Study the drawing (mm; zero at the part's minimum x, y, z) and answer. A direction names the side the tool comes from. Give positions to 0.01 mm unless a question says otherwise; leave off trailing zeros. Loops run counter-clockwise (first coordinate to the right, second up) from the corner with the lowest first, then second, coordinate; pieces in that order, holes last. Notation, with made-up numbers: M 66,-30 L 92,-30 A18 cw 92,-7 Z; hole C 33,53.25 d5. An arc over 180 degrees is marked long. Return JSON: item names as keys, results as strings.
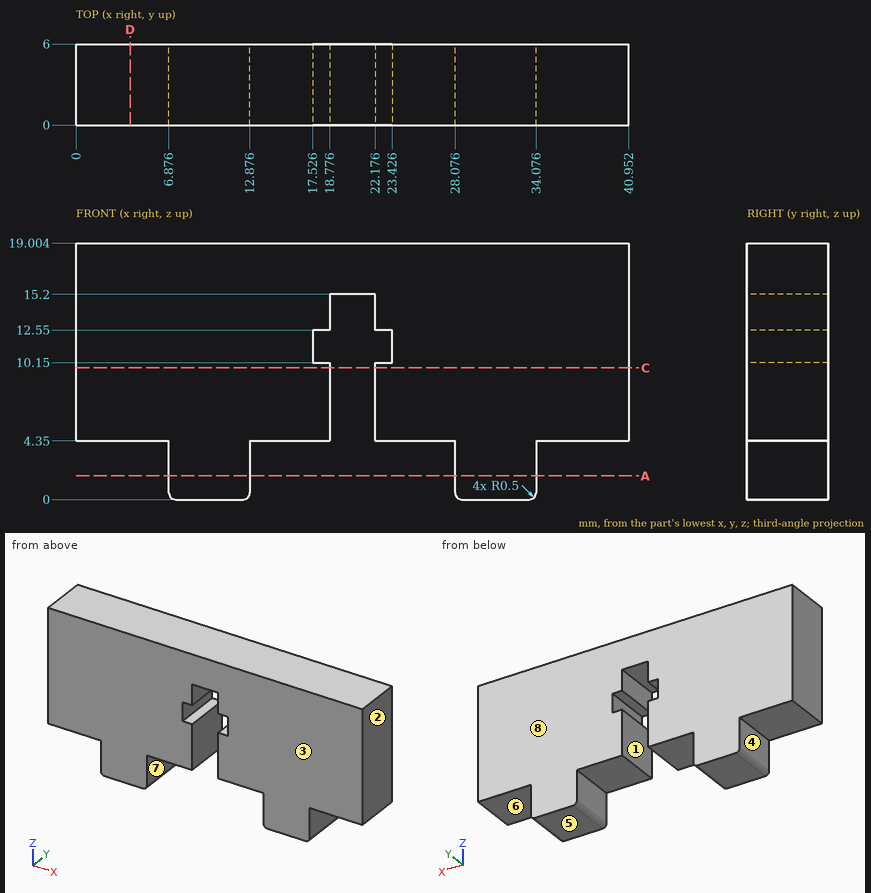
(1) The part is cut by section C-C (z = 9.75). Determine the outline of the cut face in (x, y) (1 decimal), and give its area (3 significant figures).
Values follow:
{"outline": "M 0,0 L 18.8,0 L 18.8,6 L 0,6 Z; M 22.2,0 L 41,0 L 41,6 L 22.2,6 Z", "area": "225 mm²"}
(2) Given pin 1 (1.5 mm diameter, centred on x = 5.5, z = 3, fed in from +Y); pin 2 (1.4 mm diameter, centred on x = 18, y = 2.5, fed in from -Z); pin 3 (1.2 mm diameter, centred on y = 4, z = 2, fed in from +X), each flat-ended and moving along its own axis, determine where each tip first touches the part or whether it passes through.
Values follow:
{"pin 1": "through", "pin 2": "z = 4.35", "pin 3": "x = 34.08"}
(3) A tool of negligible diameter and unlimited length cuts with its end or side. For the marked faces 4, 5, 6, 7 and 8, from which of +Z, -Z, +X, -X, +Y, -Y can it reach the whole face along a straight path? Write none if from no direction.
Values follow:
{"face 4": "-Z, -X, +Y, -Y", "face 5": "-Z, +X, -X, +Y, -Y", "face 6": "-Z, +X, +Y, -Y", "face 7": "-Z, +Y, -Y", "face 8": "+Z, -Z, +X, -X, +Y"}
(4) The part is cut by section D-D (x = 4). Determine the outline of the cut face in (y, z).
Values follow:
{"outline": "M 0,4.35 L 6,4.35 L 6,19 L 0,19 Z"}
(5) Straight lines are drawn through the part: line 1 along X through (y, z) = (1.45, 3.75) (1 decimal); line 2 along X through (y, z) = (1.5, 10.75) (1 decimal); line 3 along Z through (x, y) = (22.5, 1.25). For each, find the intervals that lie inside material, in ascending order.
Values follow:
{"line 1": "6.9 to 12.9, 28.1 to 34.1", "line 2": "0 to 17.5, 23.4 to 41", "line 3": "4.35 to 10.15, 12.55 to 19"}
(6) The part is cut by section A-A (z = 1.75). Determine the outline of the cut face in (x, y) (1 decimal).
Values follow:
{"outline": "M 6.9,0 L 12.9,0 L 12.9,6 L 6.9,6 Z; M 28.1,0 L 34.1,0 L 34.1,6 L 28.1,6 Z"}
(7) Determine the mould class of the marked faces 1, 2 and 3 for opening direction X: released by +X, released by -X, zero draft, split by the parting line, or undercut.
Values follow:
{"face 1": "undercut", "face 2": "released by +X", "face 3": "zero draft"}
